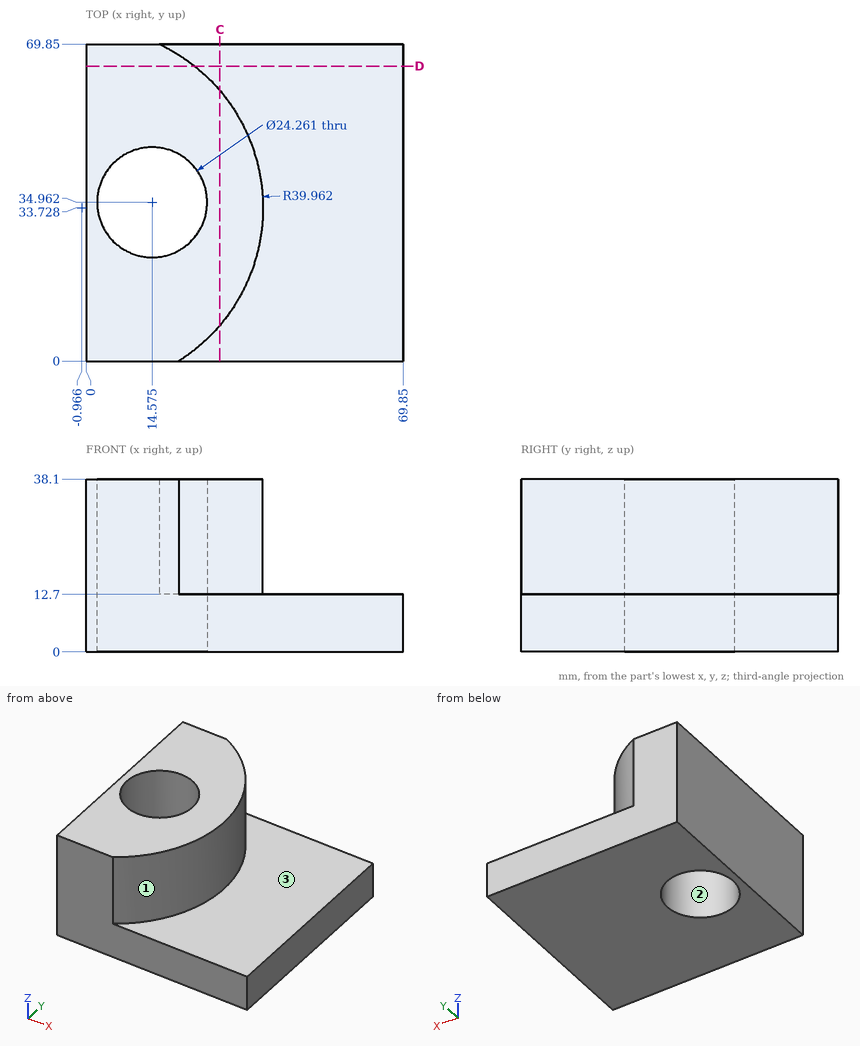
Verification items for this drawing (mm, ordinates from the low corner). Coordinates: 2 decimals unless noted, no trailing zeros. Write each loop counter-clockwise with the first axis right and the second up, starting at its lowest first coordinate (ties: lowest second). Pieces come first, ordered by that corner, then holes. Notation, with made-up numbers: M -15,-18 L 4,-18 A18 ccw 4,2 Z; hole C -39.75,-33 d2. An arc over 180 degrees is marked long. Use CSV: the item, a comma, the result in double quotes.
Q1. Section check D-D, the plane y = 65. Enter the section's corners in (x, z), and give its area (3 significant figures).
Computed values:
outline,"M 0,0 L 69.85,0 L 69.85,12.7 L 23.91,12.7 L 23.91,38.1 L 0,38.1 Z"
area,"1,490 mm²"
Q2. Go/stop test with flat-tipped pins: P1, Ø4, axis at y = 25.5, z = 25.5, coming from the +X side; P2, Ø6, axis at x = 24.5, z = 16.5, coming from the +Y side; P3, Ø1.5, axis at y = 61, z = 32, coming from the +X side (1 decimal). Record where each tip stops, or that it passes through.
Computed values:
P1,"x = 38.51"
P2,"y = 66.78"
P3,"x = 28.9"
Q3. Mould release check, pull along Y, two halves, no side actions. Record for the marked faces 1, 2 and 3: pulls with the +Y half, pulls with the -Y half, needs draft (parallel to the pull), parting line crosses it, or undercut.
Computed values:
face 1,"parting line crosses it"
face 2,"undercut"
face 3,"needs draft"
Q4. Thickness scan on line 1 along Z through (x, y) = (43, 11); line 2 along X through (y, z) = (44, 19.5) (1 decimal); line 3 along X through (y, z) = (45.5, 30.5) (1 decimal). Record the ranges inside material, lowest first. Write a range as [from, to].
Computed values:
line 1,"[0, 12.7]"
line 2,"[0, 6.5], [22.7, 37.7]"
line 3,"[0, 8.6], [20.6, 37.2]"
Q5. Section check C-C, the plane x = 29.5. Enter the section's corners in (y, z).
Computed values:
outline,"M 0,0 L 69.85,0 L 69.85,12.7 L 59.59,12.7 L 59.59,38.1 L 7.87,38.1 L 7.87,12.7 L 0,12.7 Z"
